```python
from build123d import *

# Parameters (mm, degrees)
BOSS_EXTRUDE1_START = 0.2
BOSS_EXTRUDE1_DEPTH = 9.6
SKETCH3_R           = 1.65
CUT_EXTRUDE1_DEPTH  = 5
CHAMFER1_SIZE       = 1


with BuildPart() as part:
    # Sketch2 → Boss-Extrude1 (new body)
    with BuildSketch(Plane.XZ.offset(17.988801204).offset(BOSS_EXTRUDE1_START)):
        Polygon((26.026797653, -5), (31.181498191, -5), (31.181498191, -2.5), (31.181498191, 0), (26.381498191, 0), (26.381498191, 2.5), (33.181498191, 2.5), (33.181498191, -7), (27.181498191, -7), align=None)
    extrude(amount=BOSS_EXTRUDE1_DEPTH)

    # Sketch3 → Cut-Extrude1 (cut)
    with BuildSketch(Plane.XY.offset(2.5)):
        with Locations((28.681498191, -22.988801204)):
            Circle(SKETCH3_R)
    extrude(amount=-CUT_EXTRUDE1_DEPTH, mode=Mode.SUBTRACT)

    # Chamfer1
    chamfer1_edges = [part.edges().sort_by_distance(p)[0] for p in [
        (33.181498191, -22.988801204, -7),
        (33.181498191, -22.988801204, 2.5),
    ]]
    chamfer(chamfer1_edges, length=CHAMFER1_SIZE)


solid = part.part
```
Model file for the job. Use its own axes, mm. A direction names the side the tool comes from. Give positions to 0.01 mm unless a question says otherwise; leave off trailing zeros. Write each loop counter-clockwise with the first axis right and the second up, starting at its lowest first coordinate (ties: lowest second). Pieces come first, ordered by that corner, then holes. Notation, with made-up numbers: (-34.5, 68.5) - (-3.5, 68.5) arc R29 cw to (-3.5, 106.5) - close; hole circle Ø7 at (30.5, 38). An arc over 180 degrees is marked (long way). One line per question, with ' | ' between items. Start each with the question number.
(1) Pin check, flat tip, straight feed: P1, Ø0.8, axis at y = -20.5, z = 1.5, coming from the -X side. Stop position of the tip, or through.
(2) Wall check: line 1 along Z through (x, y) = (27.25, -25.25); line 2 along X through (y, z) = (-24.75, -4.5); line 3 along Y through (x, z) = (28.75, 0.5). Give the ranges that are in metal, low to high. Write a range as from..to.
(3) Slice it at C-C on y = -25. Write the cut outline in (x, z), plus the area to 3 significant figures.
(4) Slice it at B-B on y = -21.75. Write the cut outline in (x, z), plus the area to 3 significant figures.
(5) 3-axis set-ups, long thin cutter, end or side, ignore diameter. For faces 4 (the face through (31.181, -23, -2)), 5 (the face through (32.69, -22.92, 1.99)), 6 (the face through (26.381, -23, 1)): which of +Z, -Z, +X, -X, +Y, -Y reach the whole face in a straight line?
(6) Slice it at A-A on x = 30.75. Write the cut outline in (y, z).
(7) Slice it at D-D on x = 29.25. Write the cut outline in (y, z), plus the area to 3 significant figures.
(8) Two-plate mould, pull along Z, no slides. Class faces 1 (the face through (26.61, -22.92, -6.01)), 2 (the face through (29, -23, -5)), 3 (the face through (29.443, -24.453, 1.268)): +Z half, -Z half, draft (parallel to the pull), parting line (faces both ways), or undercut.
Results below:
1) P1: x = 26.38
2) line 1: -7..-5, 0..2.5 | line 2: 31.18..33.18 | line 3: -27.79..-24.64, -21.34..-18.19
3) outline: (26.03, -5) - (27.18, -7) - (32.18, -7) - (33.18, -6) - (33.18, 1.5) - (32.18, 2.5) - (26.38, 2.5) - (26.38, 0) - (31.18, 0) - (31.18, -5) - close | area: 39.2 mm^2
4) outline: (26.03, -5) - (27.18, -7) - (32.18, -7) - (33.18, -6) - (33.18, 1.5) - (32.18, 2.5) - (29.77, 2.5) - (29.77, 0) - (31.18, 0) - (31.18, -5) - close; (26.38, 0) - (27.59, 0) - (27.59, 2.5) - (26.38, 2.5) - close | area: 33.7 mm^2
5) face 4: -X, +Y, -Y | face 5: +Z, +X, +Y, -Y | face 6: +Z, -X, +Y, -Y
6) outline: (-27.79, -7) - (-18.19, -7) - (-18.19, -5) - (-27.79, -5) - close; (-27.79, 0) - (-18.19, 0) - (-18.19, 2.5) - (-27.79, 2.5) - close
7) outline: (-27.79, -7) - (-18.19, -7) - (-18.19, -5) - (-27.79, -5) - close; (-27.79, 0) - (-24.54, 0) - (-24.54, 2.5) - (-27.79, 2.5) - close; (-21.44, 0) - (-18.19, 0) - (-18.19, 2.5) - (-21.44, 2.5) - close | area: 35.5 mm^2
8) face 1: -Z half | face 2: undercut | face 3: draft
